from build123d import *

# Parameters (mm, degrees)
F0_R     = 3.175
F0_R_2   = 2.15265
F0_R_3   = 26.7462
F1_DEPTH = 4.7625
F2_R     = 76.2
F3_R     = 3.175
F5_DEPTH = 4.7635


with BuildPart() as f1:
    # F0 (on Front) → F1 (new body)
    with BuildSketch(Plane.XZ):
        with BuildLine():
            Line((-20.125207, 63.858887), (-45.525207, 63.858887))
            Line((-45.525207, 63.858887), (-45.525207, -56.791113))
            Line((-45.525207, -56.791113), (75.124793, -56.791113))
            Line((75.124793, -56.791113), (75.124793, -31.391113))
            Line((75.124793, -31.391113), (59.224484, -10.158949))
            Line((59.224484, -10.158949), (51.176471, 15.116615))
            ThreePointArc((51.176471, 15.116615), (43.192477, 29.054031), (30.182356, 38.473821))
            ThreePointArc((30.182356, 38.473821), (27.19297, 39.642493), (24.115979, 40.55592))
            Line((24.115979, 40.55592), (-0.834672, 46.834476))
            Line((-0.834672, 46.834476), (-20.125207, 63.858887))
        make_face()
        with Locations((-32.825207, -44.091113)):
            Circle(F0_R, mode=Mode.SUBTRACT)
        with Locations((6.910989, -25.907532)):
            Circle(F0_R_2, mode=Mode.SUBTRACT)
        with Locations((-14.641626, -4.354918)):
            Circle(F0_R_2, mode=Mode.SUBTRACT)
        with Locations((17.974793, -44.091113)):
            Circle(F0_R, mode=Mode.SUBTRACT)
        with Locations((43.374793, -44.091113)):
            Circle(F0_R, mode=Mode.SUBTRACT)
        with Locations((68.774793, -44.091113)):
            Circle(F0_R, mode=Mode.SUBTRACT)
        with Locations((36.352408, -18.018728)):
            Circle(F0_R_2, mode=Mode.SUBTRACT)
        with Locations((-32.825207, 6.708887)):
            Circle(F0_R, mode=Mode.SUBTRACT)
        with Locations((-32.825207, 32.108887)):
            Circle(F0_R, mode=Mode.SUBTRACT)
        with Locations((-6.752821, 25.086501)):
            Circle(F0_R_2, mode=Mode.SUBTRACT)
        with Locations((-32.825207, 57.508887)):
            Circle(F0_R, mode=Mode.SUBTRACT)
        with Locations((14.799793, 3.533887)):
            Circle(F0_R_3, mode=Mode.SUBTRACT)
        with Locations((44.241213, 11.422691)):
            Circle(F0_R_2, mode=Mode.SUBTRACT)
        with Locations((22.688598, 32.975306)):
            Circle(F0_R_2, mode=Mode.SUBTRACT)
    extrude(amount=F1_DEPTH)

    # F2
    f2_edges = [f1.edges().sort_by_distance(p)[0] for p in [
        (-0.834672, -2.38125, 46.834476),
        (59.224484, -2.38125, -10.158949),
    ]]
    fillet(f2_edges, radius=F2_R)

    # F3
    f3_edges = [f1.edges().sort_by_distance(p)[0] for p in [
        (-45.525207, -2.38125, 63.858887),
        (-20.125207, -2.38125, 63.858887),
        (-45.525207, -2.38125, -56.791113),
        (75.124793, -2.38125, -31.391113),
        (75.124793, -2.38125, -56.791113),
    ]]
    fillet(f3_edges, radius=F3_R)

    # F4 (on face) → F5 (cut, through all)
    with BuildSketch(Plane.XZ.offset(4.7625)):
        with BuildLine():
            ThreePointArc((-12.90503, 29.799168), (-12.06269, 32.408274), (-13.566624, 34.700687))
            ThreePointArc((-13.566624, 34.700687), (-17.547135, 37.243821), (-21.396672, 39.981165))
            ThreePointArc((-21.396672, 39.981165), (-24.720929, 40.279463), (-26.475207, 37.440066))
            Line((-26.475207, 37.440066), (-26.475207, 19.605966))
            ThreePointArc((-26.475207, 19.605966), (-23.929722, 16.494), (-20.374838, 18.371931))
            ThreePointArc((-20.374838, 18.371931), (-17.154892, 24.422169), (-12.90503, 29.799168))
        make_face()
        with BuildLine():
            ThreePointArc((-26.475207, -34.566113), (-25.545271, -36.811177), (-23.300207, -37.741113))
            Line((-23.300207, -37.741113), (-1.272286, -37.741113))
            ThreePointArc((-1.272286, -37.741113), (1.83968, -35.195629), (-0.038251, -31.640745))
            ThreePointArc((-0.038251, -31.640745), (-12.194856, -23.460763), (-20.374838, -11.304157))
            ThreePointArc((-20.374838, -11.304157), (-23.929722, -9.426226), (-26.475207, -12.538193))
            Line((-26.475207, -12.538193), (-26.475207, -34.566113))
        make_face()
        with BuildLine():
            Line((52.277549, -32.662938), (51.688182, -31.875938))
            ThreePointArc((51.688182, -31.875938), (49.023348, -28.132604), (46.542146, -24.265108))
            ThreePointArc((46.542146, -24.265108), (44.219215, -22.76363), (41.600324, -23.653496))
            ThreePointArc((41.600324, -23.653496), (35.998656, -28.215609), (29.637837, -31.640745))
            ThreePointArc((29.637837, -31.640745), (27.759907, -35.195629), (30.871873, -37.741113))
            Line((30.871873, -37.741113), (49.736182, -37.741113))
            ThreePointArc((49.736182, -37.741113), (52.575478, -35.987036), (52.277549, -32.662938))
        make_face()
    extrude(amount=-F5_DEPTH, mode=Mode.SUBTRACT)


solid = f1.part
Read the model definition and answer for the solid it produces. Units are mm, in the model's axes. A direction names the side the tool comes from. Coordinates: 2 decimals unless noted, no trailing zeros. Order: outer loops, then holes, each group sorted by start corner. A loop starts at its lowest first (then second) coordinate and runs counter-clockwise, first axis right, second up. Notation, with made-up numbers: (11.25, 87.25) -> (19.25, 87.25) arc R6 cw to (19.25, 97.25) -> close; hole circle Ø1 at (-7.5, 51.25). An arc over 180 degrees is marked (long way). Answer as a JSON object with one key per item and string values.
1) Each of these flat-tipped pins is pushed along its axis until it touches: pin 1 (1.4 mm diameter, centred on y = -3.5, z = -20, fed in from +X); pin 2 (2 mm diameter, centred on x = 30.5, y = -0.5, fed in from +Z); pin 3 (4 mm diameter, centred on x = -14.64, z = -4.35, fed in from -Y); pin 4 (2 mm diameter, centred on y = -3.5, z = -27.5, fed in from +X). Where does it stop, or does it pass through?
Model answer:
{"pin 1": "stops at x = 67.12", "pin 2": "stops at z = 38.77", "pin 3": "passes through", "pin 4": "stops at x = 72.96"}
2) A cutting plane is placed at B-B, the plane z = 46. Determine the outline of the cut face in (x, y), plus the area to 3 significant figures.
Model answer:
{"outline": "(-45.53, -4.76) -> (6.11, -4.76) -> (6.11, 0) -> (-45.53, 0) -> close", "area": "246 mm²"}
3) A tool of negligible diameter and unlimited length cuts with its end or side. For faces 1 (the face through (36.08, -2.41, -28.16)), 2 (the face through (74.17, -2.415, -55.886)), from which of +Z, -Z, +X, -X, +Y, -Y can it reach the whole face along a straight path? Write none if from no direction.
Model answer:
{"face 1": "+Y, -Y", "face 2": "-Z, +X, +Y, -Y"}
4) Consider line 1 along Z through (x, y) = (-32.5, -3.65); line 2 along X through (y, z) = (-0.4, -17); line 3 along Z through (x, y) = (8, -1.35). Determine where each line is inside the solid, lowest interval first. Write a range as from..to.
Model answer:
{"line 1": "z = -56.79..-47.25, -40.93..3.55, 9.87..28.95, 35.27..54.35, 60.67..63.86", "line 2": "x = -45.53..-26.48, -17.38..-2.34, 31.94..34.46, 38.25..64.49", "line 3": "z = -56.79..-27.76, -24.05..-22.33, 29.4..45.23"}
5) The mould has two halves that part along X. Classify faces 3 (the face through (-12, -2, -37.741)), 4 (the face through (53.278, -2.348, 8.517)), 5 (the face through (-32, -2, 63.859)): released by +X, released by -X, zero draft, split by the parting line, or undercut.
Model answer:
{"face 3": "undercut", "face 4": "released by +X", "face 5": "zero draft"}
6) A cutting plane is placed at A-A, the plane y = -0.8. State how many separate pieces and enclosed holes the cut face has, plus the area to 3 significant figures.
Model answer:
{"separate pieces": "1", "enclosed holes": "17", "area": "7,740 mm²"}
